from build123d import *

# Parameters (mm, degrees)
SKETCH_1_W               = 20
SKETCH_1_H               = 20
EXTRUDE_1_DEPTH          = 50
SKETCH_2_R               = 2.5
CUT_EXTRUDE_1_DEPTH      = 52.961524227
PATTERN_CIRCULAR_1_COUNT = 4
FILLET_1_R               = 2


with BuildPart() as part:
    # 草图1 → 凸台-拉伸1 (new body)
    with BuildSketch(Plane.XY):
        Rectangle(SKETCH_1_W, SKETCH_1_H)
    extrude(amount=EXTRUDE_1_DEPTH)

    # 草图2 → 切除-拉伸1 (cut, through all)
    with BuildSketch(Plane.XY.offset(50)):
        Polygon((-9.1, -3.1), (-8.2, -3.1), (-8.2, -5.45), (-6.35, -5.45), (-3.5, -2.6), (-3.5, 2.6), (-6.35, 5.45), (-8.2, 5.45), (-8.2, 3.1), (-9.1, 3.1), (-9.1, 3.6), (-10, 3.6), (-10, -3.6), (-9.1, -3.6), align=None)
        Circle(SKETCH_2_R)
    cut_extrude_1 = extrude(amount=-CUT_EXTRUDE_1_DEPTH, mode=Mode.SUBTRACT)

    # 阵列(圆周)1: 切除-拉伸1 ×4 about axis
    pattern_circular_1_axis = Axis((0, 0, 0), (0, 0, 1))
    for i in range(1, PATTERN_CIRCULAR_1_COUNT):
        add(cut_extrude_1.rotate(pattern_circular_1_axis, i * 360 / PATTERN_CIRCULAR_1_COUNT), mode=Mode.SUBTRACT)

    # 圆角1
    fillet_1_edges = [part.edges().sort_by_distance(p)[0] for p in [
        (10, -10, 25),
        (-10, -10, 25),
        (-10, 10, 25),
        (10, 10, 25),
    ]]
    fillet(fillet_1_edges, radius=FILLET_1_R)


solid = part.part
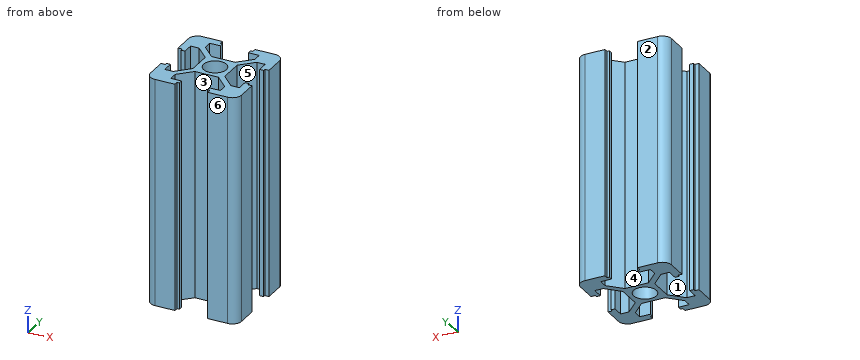
Can you work these out from the model? Positions are in its coordinate system, mm. Face numbers are marked on the shaded views. A direction names the side the tool comes from. Coordinates: 2 decimals unless noted, no trailing zeros. Write each loop counter-clockwise with the first axis right and the second up, starting at its lowest first coordinate (ties: lowest second). Pieces come first, ordered by that corner, then holes. Notation, with made-up numbers: (76.5, -25.5) -> (98.5, -25.5) arc R14 cw to (98.5, -17.5) -> close; hole circle Ø11 at (29, -29.75). An arc over 180 degrees is marked (long way). Write each question's results on one line, items separated by ' | '. Start each with the question number.
Item 1: Thinking about a two-plate mould opening in Y: for the marked faces 4, 5 and 6, which applies, released by +Y, released by -Y, zero draft, split by the parting line, or undercut?
Item 2: I'm going to push flat-ended pins straight in: P1, Ø1.5, axis at y = 1.5, z = 25.5, coming from the -X side; P2, Ø1, axis at x = 9, z = 24, coming from the +Y side; P3, Ø4, axis at y = 1, z = 22.5, coming from the +X side. Where does each tip first touch, or does it pass through?
Item 3: Please list where these lines run through material, in increasing order: probe 1 along X at (y, z) = (-6.75, 45); probe 2 along Y at (x, z) = (0, 34); probe 3 along Y at (x, z) = (-4.25, 25).
Item 4: On a 3-axis mill with a long thin cutter (end or side, diameter ignored), from which of +Z, -Z, +X, -X, +Y, -Y can I reach the whole of each face in a straight line? I mean the marked faces 1, 2 and 3. Say none if no direction works.
Item 5: If we section it at A-A, the plane y = 0: Write out the boundary of the cut face in (x, z).
Answer block:
1) face 4: released by +Y | face 5: undercut | face 6: released by -Y
2) P1: x = -3.5 | P2: y = 9.94 | P3: x = 3.9
3) probe 1: -10 to -5.45, 5.45 to 10 | probe 2: -3.5 to -2.5, 2.5 to 3.5 | probe 3: -10 to -8.2, -5.15 to -3.35, 3.35 to 5.15, 8.2 to 10
4) face 1: +Z, -Z | face 2: +Z, -Z, +X, -X, +Y | face 3: +Z, -Z, -Y
5) outline: (-3.5, 0) -> (-2.5, 0) -> (-2.5, 50) -> (-3.5, 50) -> close; (2.5, 0) -> (3.5, 0) -> (3.5, 50) -> (2.5, 50) -> close
